Can you work these out from the model? Positions are in its coordinate system, mm. A direction names the side the tool comes from. Round coordinates to 2 decimals unless told otherwise and drop trailing zeros. Loops run counter-clockwise (first coordinate to the right, second up) from the corner with the lowest first, then second, coordinate; pieces in that order, holes last. Notation, with made-up numbers: M 1,57.5 L 52,57.5 A22 ccw 52,89.5 Z; hole C -30.75,16.25 d10. An arc over 180 degrees is marked long. Use a Markdown table: item, result. Add a question column.
```python
from build123d import *

# Parameters (mm, degrees)
F0_W     = 508
F0_H     = 304.8
F1_DEPTH = 9.525
F3_DEPTH = 19.05
F5_DEPTH = 19.05


# Not quite as in the source:
# - a feature names something its author has since deleted; it is built from what else it names


with BuildPart() as f1:
    # F0 (on Front) → F1 (new body, symmetric)
    with BuildSketch(Plane.XZ):
        Rectangle(F0_W, F0_H)
    extrude(amount=F1_DEPTH, both=True)

    # F2 (on face) → F3 (cut)
    with BuildSketch(Plane(origin=(-254, 0, 0), x_dir=(0, -1, 0), z_dir=(-1, 0, 0))):
        Polygon((-9.525, 128.2455678842), (9.525, 133.35), (9.525, 152.4), (-9.525, 152.4), align=None)
        Polygon((9.525, 38.1), (9.525, 57.15), (-9.525, 62.2544321158), (-9.525, 32.9955678842), align=None)
        Polygon((9.525, -57.15), (9.525, -38.1), (-9.525, -32.9955678842), (-9.525, -62.2544321158), align=None)
        Polygon((9.525, -152.4), (9.525, -133.35), (-9.525, -128.2455678842), (-9.525, -152.4), align=None)
    extrude(amount=-F3_DEPTH, mode=Mode.SUBTRACT)

    # F4 (on face) → F5 (cut)
    with BuildSketch(Plane.YZ.offset(254)):
        Polygon((-9.525, 132.499261314), (9.525, 127.3948291982), (9.525, 152.4), (-9.525, 152.4), align=None)
        Polygon((9.525, 32.1448291982), (9.525, 63.1051708018), (-9.525, 58.000738686), (-9.525, 37.249261314), align=None)
        Polygon((9.525, -63.1051708018), (9.525, -32.1448291982), (-9.525, -37.249261314), (-9.525, -58.000738686), align=None)
        Polygon((9.525, -152.4), (9.525, -127.3948291982), (-9.525, -132.499261314), (-9.525, -152.4), align=None)
    extrude(amount=-F5_DEPTH, mode=Mode.SUBTRACT)


solid = f1.part
```
(1) Suppose I cut it at A-A on y = 1.75. List the corners of the cut face in (x, z) for me.
(2) If I drill on probe 1 along X at (y, z) = (8.25, 42.5), over which ranges is the centre line in solid material (lowest first)? Write a range as [from, to].
(3) On a 3-axis mill with a long thin cutter (end or side, diameter ignored), from which of +Z, -Z, +X, -X, +Y, -Y can I reach the whole of each face in a straight line? I mean faces 4 (the face through (234.95, 0, -140)), 5 (the face through (-244.608, 0.133, 35.512)), 6 (the face through (244.61, -0.13, 129.98)), 7 (the face through (-244.608, -0.133, -130.834)). Say none if no direction works.
(4) Thinking about a two-plate mould opening in Z: for faces 1 (the face through (244.608, 0.133, -129.911)), 2 (the face through (244.61, -0.13, -60.52)), 3 (the face through (-244.608, 0.133, 130.762)), which applies, released by +Z, released by -Z, zero draft, split by the parting line, or undercut?
(5) I'm going to push flat-ended pins straight in: pin 1 (5.5 mm diameter, centred on y = -3, z = -136.5, fed in from +X); pin 2 (9.5 mm diameter, centred on y = 2.5, z = 137, fed in from -X). Where does each tip first touch, or does it pass through?
Results below:
| question | item | result |
|---|---|---|
| 1 | outline | M -254,-130.33 L -234.95,-130.33 L -234.95,-152.4 L 234.95,-152.4 L 234.95,-129.48 L 254,-129.48 L 254,-61.02 L 234.95,-61.02 L 234.95,-34.23 L 254,-34.23 L 254,34.23 L 234.95,34.23 L 234.95,61.02 L 254,61.02 L 254,129.48 L 234.95,129.48 L 234.95,152.4 L -234.95,152.4 L -234.95,130.33 L -254,130.33 L -254,60.17 L -234.95,60.17 L -234.95,35.08 L -254,35.08 L -254,-35.08 L -234.95,-35.08 L -234.95,-60.17 L -254,-60.17 Z |
| 2 | probe 1 | x = [-234.95, 234.95] |
| 3 | face 4 | -Z, +X, +Y |
| 3 | face 5 | -X, +Y |
| 3 | face 6 | +Z, +X, +Y |
| 3 | face 7 | -Z, -X, +Y |
| 4 | face 1 | released by -Z |
| 4 | face 2 | undercut |
| 4 | face 3 | released by +Z |
| 5 | pin 1 | stops at x = 234.95 |
| 5 | pin 2 | stops at x = -234.95 |
